```python
from build123d import *

# Parameters (mm, degrees)
F1_DEPTH = 150
F2_R     = 5
F3_DEPTH = 19.900416
F4_W     = 100
F4_H     = 20
F5_DEPTH = 19.900416


with BuildPart() as f1:
    # F0 (on Front) → F1 (new body)
    with BuildSketch(Plane.XZ):
        Polygon((75, 90), (55.100584, 90), (55.100584, 10), (-24.899416, 10), (-24.899416, -40.001069), (-75, -40.001069), (-75, -90), (75, -90), align=None)
    extrude(amount=F1_DEPTH)

    # F2 (on face) → F3 (cut, through all)
    with BuildSketch(Plane(origin=(55.100584, 0, 0), x_dir=(0, -1, 0), z_dir=(-1, 0, 0))):
        with Locations((82.543276, 70)):
            Circle(F2_R)
    extrude(amount=-F3_DEPTH, mode=Mode.SUBTRACT)

    # F4 (on face) → F5 (cut, through all)
    with BuildSketch(Plane(origin=(55.100584, 0, 0), x_dir=(0, -1, 0), z_dir=(-1, 0, 0))):
        with Locations((81.568733, 39.006799)):
            Rectangle(F4_W, F4_H)
    extrude(amount=-F5_DEPTH, mode=Mode.SUBTRACT)


solid = f1.part
```
Check sheet for the modelled part. Datum: model origin and axes. Units: mm. A direction names the side the tool comes from. Give positions to 0.01 mm unless a question says otherwise; leave off trailing zeros. Write each loop counter-clockwise with the first axis right and the second up, starting at its lowest first coordinate (ties: lowest second). Pieces come first, ordered by that corner, then holes. Notation, with made-up numbers: (63.25, -13.75) - (110.25, -13.75) arc R26 cw to (110.25, 7.25) - close; hole circle Ø9 at (5, -10.75). An arc over 180 degrees is marked (long way). Answer as a JSON object with one key per item and string values. Group by question number.
1) Release check for a two-part mould opening along Z. For faces 4 (the face through (75, -74, -1)), 5 (the face through (-50, -74, -40.001)), 6 (the face through (64.91, -87.16, 68.08)) record: pulls with the +Z half, pulls with the -Z half, needs draft (parallel to the pull), parting line crosses it, or undercut.
2) Thickness scan on probe 1 along Y at (x, z) = (61, 35.5); probe 2 along Y at (x, z) = (59, 70.5); probe 3 along X at (y, z) = (-85.5, 6.5). Record the ranges inside material, lowest first. Write a range as from..to.
3) Sectioned sample at A-A (y = -60.5). Record the cut outline in (x, z), then the cut area to 3 significant figures.
4) Sectioned sample at B-B (z = 70). Record the cut outline in (x, y).
5) Sectioned sample at C-C (x = 64). Record the cut outline in (y, z).
6) Access from +Z, -Z, +X, -X, +Y, -Y to the whole of each face (thin tool, end or side, straight path). Record for faces 1 (the face through (16, -74, 10)), 2 (the face through (65, -74, 90)), 3 (the face through (65, -31.569, 39)).
7) Depth check by flat-ended pin: P1, Ø22, axis at x = 67.5, z = 44, coming from the +Y side; P2, Ø15, axis at y = -98.5, z = -13.5, coming from the -X side; P3, Ø6, axis at x = -26.5, y = -79.5, coming from the +Z side; P4, Ø24, axis at y = -101.5, z = 48.5, coming from the -X side. Enter the tip coordinate at first touch or a pass-through.
8) Sectioned sample at D-D (x = -48). Record the cut outline in (y, z).
Geometry results:
{
 "1": {"face 4": "needs draft", "face 5": "pulls with the +Z half", "face 6": "undercut"},
 "2": {"probe 1": "y = -150..-131.57, -31.57..0", "probe 2": "y = -150..-87.52, -77.57..0", "probe 3": "x = -24.9..75"},
 "3": {"outline": "(-75, -90) - (75, -90) - (75, 29.01) - (55.1, 29.01) - (55.1, 10) - (-24.9, 10) - (-24.9, -40) - (-75, -40) - close; (55.1, 49.01) - (75, 49.01) - (75, 90) - (55.1, 90) - close", "area": "13,700 mm^2"},
 "4": {"outline": "(55.1, -150) - (75, -150) - (75, -87.54) - (55.1, -87.54) - close; (55.1, -77.54) - (75, -77.54) - (75, 0) - (55.1, 0) - close"},
 "5": {"outline": "(-150, -90) - (0, -90) - (0, 90) - (-150, 90) - close; hole (-131.57, 29.01) - (-31.57, 29.01) - (-31.57, 49.01) - (-131.57, 49.01) - close; hole circle Ø10 at (-82.54, 70)"},
 "6": {"face 1": "+Z, -X, +Y, -Y", "face 2": "+Z, +X, -X, +Y, -Y", "face 3": "+X, -X"},
 "7": {"P1": "stops at y = 0", "P2": "stops at x = -24.9", "P3": "stops at z = 10", "P4": "stops at x = 55.1"},
 "8": {"outline": "(-150, -90) - (0, -90) - (0, -40) - (-150, -40) - close"}
}
